Could you check a few things on this model? Use its own coordinates, in mm. A direction names the side the tool comes from. Coordinates: 2 decimals unless noted, no trailing zeros. Order: outer loops, then holes, each group sorted by start corner. A loop starts at its lowest first (then second) coordinate and runs counter-clockwise, first axis right, second up. Notation, with made-up numbers: (4.5, 88.5) -> (38.5, 88.5) arc R8 cw to (38.5, 101.5) -> close; hole circle Ø3 at (-19.5, -31.75). An arc over 180 degrees is marked (long way). Use a Markdown table: item, result. Add a question column.
1) If we section it at B-B (x = 1128.5): Write out the boundary of the cut face in (y, z).
2) If we section it at D-D (x = 170): Write out the boundary of the cut face in (y, z).
3) Which directions (+Z, -Z, +X, -X, +Y, -Y) give clear straight access to the entire face, cutting with the end or side of a thin tool? Please do faces 1 (the flat face through (1038, 438, 200)), 2 (the flat face through (652.086, 437.058, 98.635)), 3 (the flat face through (1439.703, 431.71, 98.6)).
4) Thinking about a two-plate mould opening in X: for faces 4 (the flat face through (2294, 99, 321)), 5 (the flat face through (1027, 265, 0)), 6 (the flat face through (1039, 437, 197.5)), which applies, +X half, -X half, draft (parallel to the pull), parting line (faces both ways), or undercut?
5) If we section it at C-C (z = 309.5): Write out the boundary of the cut face in (x, y), plus the area to 3 significant figures.
6) If we section it at A-A (y = 43): Write out the boundary of the cut face in (x, z).
7) If I drill on L1, parallel to Z at x = 909, y = 462; L2, parallel to Z at x = 24, y = 62, over which ranges is the centre line in solid material (lowest first)? Write a range as [from, to].
8) Will these pins go through, and if not, where does the flat tip stop? pin 1 Ø3 at (y, z) = (68.5, 150.5) entering from -X; pin 2 Ø2 at (x, z) = (1521.5, 177) entering from +Y.
```python
from build123d import *

# Parameters (mm, degrees)
F1_DEPTH      = 200
F2_W          = 200
F2_H          = 240
F3_DEPTH      = 2294
F3_DEPTH_BACK = 206
F4_T          = -2.5


with BuildPart() as f1:
    # F0 (on Top) → F1 (new body)
    with BuildSketch(Plane.XY):
        Polygon((-205.6466794014, 200), (-205.6466794014, 0), (2294.3533205986, 0), (2294.3533205986, 200), (1464.3533205986, 200), (1044.3533205986, 200), (624.3533205986, 200), align=None)
        Polygon((674.3533205986, 670), (624.3533205986, 200), (1044.3533205986, 200), (1044.3533205986, 670), align=None)
        Polygon((1044.3533205986, 200), (1464.3533205986, 200), (1414.3533205986, 670), (1044.3533205986, 670), align=None)
    extrude(amount=F1_DEPTH)

    # F2 (on Right) → F3 (join, two sides)
    with BuildSketch(Plane.YZ) as f3_sk:
        with Locations((100, 319.0685760975)):
            Rectangle(F2_W, F2_H)
    extrude(amount=F3_DEPTH)
    extrude(f3_sk.sketch, amount=-F3_DEPTH_BACK)

    # F4
    f4_openings = [f1.faces().sort_by_distance(p)[0] for p in [
        (1044.353321, 670, 100),
    ]]
    offset(amount=F4_T, openings=f4_openings, kind=Kind.INTERSECTION)


solid = f1.part
```
Answer sheet:
| question | item | result |
|---|---|---|
| 1 | outline | (0, 0) -> (670, 0) -> (670, 2.5) -> (2.5, 2.5) -> (2.5, 436.57) -> (197.5, 436.57) -> (197.5, 197.5) -> (670, 197.5) -> (670, 200) -> (200, 200) -> (200, 439.07) -> (0, 439.07) -> close |
| 2 | outline | (0, 0) -> (200, 0) -> (200, 439.07) -> (0, 439.07) -> close; hole (2.5, 2.5) -> (197.5, 2.5) -> (197.5, 436.57) -> (2.5, 436.57) -> close |
| 3 | face 1 | +Z, +X, -X, +Y |
| 3 | face 2 | none |
| 3 | face 3 | +Z, -Z, +X, +Y |
| 4 | face 4 | +X half |
| 4 | face 5 | draft |
| 4 | face 6 | undercut |
| 5 | outline | (-206, 0) -> (2294, 0) -> (2294, 200) -> (-206, 200) -> close; hole (-203.5, 2.5) -> (2291.5, 2.5) -> (2291.5, 197.5) -> (-203.5, 197.5) -> close |
| 5 | area | 13,500 mm2 |
| 6 | outline | (-206, 199.07) -> (-205.65, 199.07) -> (-205.65, 0) -> (2294.35, 0) -> (2294.35, 200) -> (2294, 200) -> (2294, 439.07) -> (-206, 439.07) -> close; hole (-203.5, 201.57) -> (-203.15, 201.57) -> (-203.15, 2.5) -> (2291.85, 2.5) -> (2291.85, 197.5) -> (2291.5, 197.5) -> (2291.5, 436.57) -> (-203.5, 436.57) -> close |
| 7 | L1 | [0, 2.5], [197.5, 200] |
| 7 | L2 | [0, 2.5], [436.57, 439.07] |
| 8 | pin 1 | x = -205.65 |
| 8 | pin 2 | y = 200 |
